Geometry check sheet. Reference: the model listing, model coordinates, mm. A direction names the side the tool comes from. Give positions to 0.01 mm unless a question says otherwise; leave off trailing zeros. Loops run counter-clockwise (first coordinate to the right, second up) from the corner with the lowest first, then second, coordinate; pieces in that order, holes last. Notation, with made-up numbers: (46.25, -18) - (54.25, -18) arc R7 ccw to (54.25, -8) - close; hole circle Ø7 at (-12.5, 13.5). An arc over 180 degrees is marked (long way). Write item = value, one per line. Start each with the question number.
from build123d import *

# Parameters (mm, degrees)
CUT_EXTRUDE1_DEPTH = 1.5


with BuildPart() as part:
    # Sketch1 → Revolve1 (revolve)
    with BuildSketch(Plane(origin=(0, 0, 0), x_dir=(0, 0, -1), z_dir=(1, 0, 0)), mode=Mode.PRIVATE) as revolve1_sk:
        Polygon((-1.7, 0), (-1.7, 3), (-1.49, 3), (0, 1.51), (0, 1.5), (10.3, 1.5), (10.3, 0), align=None)
    revolve(revolve1_sk.sketch.rotate(Axis((0, 0, 5.584882278), (0, 0, -1)), 180), axis=Axis((0, 0, 5.584882278), (0, 0, -1)))

    # Sketch2 → Cut-Extrude1 (cut)
    with BuildSketch(Plane.XY.offset(1.7)):
        Polygon((0.577350269, -1), (1.154700538, 0), (0.577350269, 1), (-0.577350269, 1), (-1.154700538, 0), (-0.577350269, -1), align=None)
    extrude(amount=-CUT_EXTRUDE1_DEPTH, mode=Mode.SUBTRACT)


solid = part.part
1) Cross-section at C-C on z = -9. Enter the section's corners in (x, y), and give its area (3 significant figures).
2) Material ranges on line 1 along Z through (x, y) = (-0.5, 0); line 2 along Y through (x, z) = (-0.1, -5.25); line 3 along Y through (x, z) = (0.8, -3.25), recorded low to high.
3) Tool access check on faces 1 (the face through (0, 0, -10.3)), 2 (the face through (0, 0, 0.2)). Record the directions out of +Z, -Z, +X, -X, +Y, -Y that give a thin tool (end or side, any length) a straight path to the whole face; none if there is none.
4) Release check for a two-part mould opening along Y. For faces 3 (the face through (-0.45, -1.43, -5.22)), 4 (the face through (0, 1.3, 1.7)), 5 (the face through (0.87, 0.49, 0.96)) record: pulls with the +Y half, pulls with the -Y half, needs draft (parallel to the pull), parting line crosses it, or undercut.
5) Cross-section at A-A on z = 1. Enter the section's corners in (x, y), and give its area (3 significant figures).
6) Gauge pin test, flat ends, axial feed: P1, Ø0.6, axis at x = 0, z = 1, coming from the -Y side; P2, Ø0.6, axis at x = 0, y = 0.5, coming from the +Z side; P3, Ø2, axis at x = 0.5, z = 0, coming from the +Y side. Record the tip position at first contact, or that the pin passes through.
Checked values:
q1.outline = circle Ø3 at (0, 0)
q1.area = 7.07 mm²
q2.line_1 = -10.3 to 0.2
q2.line_2 = -1.5 to 1.5
q2.line_3 = -1.27 to 1.27
q3.face_1 = -Z, +X, -X, +Y, -Y
q3.face_2 = +Z
q4.face_3 = parting line crosses it
q4.face_4 = needs draft
q4.face_5 = undercut
q5.outline = circle Ø5.02 at (0, 0); hole (-1.15, 0) - (-0.58, -1) - (0.58, -1) - (1.15, 0) - (0.58, 1) - (-0.58, 1) - close
q5.area = 16.3 mm²
q6.P1 = -2.81
q6.P2 = 0.2
q6.P3 = 2.47
